Check sheet for the modelled part. Datum: model origin and axes. Units: mm. A direction names the side the tool comes from. Round coordinates to 2 decimals unless told otherwise and drop trailing zeros. Loops run counter-clockwise (first coordinate to the right, second up) from the corner with the lowest first, then second, coordinate; pieces in that order, holes last. Notation, with made-up numbers: (81, 15) - (138, 15) arc R28 ccw to (138, 42) - close; hole circle Ø4 at (79, 45.25). An arc over 180 degrees is marked (long way). Put each result on its own line as item: value.
```python
from build123d import *

# Parameters (mm, degrees)
ESQUISSE1_R             = 7.366
BOSS_EXTRU_1_DEPTH      = 9.398
BOSS_EXTRU_2_START      = -2.1844
BOSS_EXTRU_2_DEPTH      = 2.1844
CONG_1_R                = 2.54
ESQUISSE3_R             = 1.143
ENL_V_MAT_EXTRU_2_DEPTH = 16.678200152


with BuildPart() as part:
    # Esquisse1 → Boss.-Extru.1 (new body)
    with BuildSketch(Plane.XY):
        Circle(ESQUISSE1_R)
    extrude(amount=BOSS_EXTRU_1_DEPTH)

    # Esquisse2 → Boss.-Extru.2 (add)
    with BuildSketch(Plane.XY.offset(9.398).offset(BOSS_EXTRU_2_START)):
        with BuildLine():
            Line((7.366, 2.794), (6.815535195, 2.794))
            ThreePointArc((6.815535195, 2.794), (7.22707369, 1.423854584), (7.366, 0))
            Line((7.366, 0), (10.16, 0))
            ThreePointArc((10.16, 0), (9.341656347, 1.975656347), (7.366, 2.794))
        make_face()
        with BuildLine():
            Line((10.16, 0), (7.366, 0))
            ThreePointArc((7.366, 0), (7.22707369, -1.423854584), (6.815535195, -2.794))
            Line((6.815535195, -2.794), (7.366, -2.794))
            ThreePointArc((7.366, -2.794), (9.341656347, -1.975656347), (10.16, 0))
        make_face()
        with BuildLine():
            Line((-7.366, 0), (-10.16, 0))
            ThreePointArc((-10.16, 0), (-9.341656347, -1.975656347), (-7.366, -2.794))
            Line((-7.366, -2.794), (-6.815535195, -2.794))
            ThreePointArc((-6.815535195, -2.794), (-7.22707369, -1.423854584), (-7.366, 0))
        make_face()
        with BuildLine():
            Line((-6.815535195, 2.794), (-7.366, 2.794))
            ThreePointArc((-7.366, 2.794), (-9.341656347, 1.975656347), (-10.16, 0))
            Line((-10.16, 0), (-7.366, 0))
            ThreePointArc((-7.366, 0), (-7.22707369, 1.423854584), (-6.815535195, 2.794))
        make_face()
    extrude(amount=BOSS_EXTRU_2_DEPTH)

    # Congé1
    # the kernel refuses this fillet: 2.54 mm, written as the material it adds along each edge
    with BuildSketch(Plane(origin=(6.815535195, 2.794, 7.2136), x_dir=(-0.45524151464262924, 0.8903679932173465, 0), z_dir=(0, 0, 1)), Plane(origin=(-6.815535195, -2.794, 7.2136), x_dir=(0.4552415146426176, -0.8903679932173524, 0), z_dir=(0, 0, 1))) as cong_1_piece_1:
        with BuildLine():
            CenterArc((1.442130851, -2.531130754), CONG_1_R, 94.789504406, 46.813825589)
            Line((-0.548542223, -0.953531086), (-0.74760953, -0.795771119))
            ThreePointArc((-0.74760953, -0.795771119), (-0.476747902, -0.374484899), (-0.22615347, 0.115631345))
            Line((-0.22615347, 0.115631345), (0.021207807, 0.253113075))
            ThreePointArc((0.021207807, 0.253113075), (0.615026392, 0.228279187), (1.208844978, 0.253113075))
            Line((1.208844978, 0.253113075), (1.230052785, 0))
        make_face()
    extrude(amount=2.1844)
    with BuildSketch(Plane(origin=(6.815535195, -2.794, 7.2136), x_dir=(-0.4552415146426287, -0.8903679932173468, 0), z_dir=(0, 0, 1)), Plane(origin=(-6.815535195, 2.794, 7.2136), x_dir=(0.45524151464261825, 0.890367993217352, 0), z_dir=(0, 0, 1))) as cong_1_piece_2:
        with BuildLine():
            CenterArc((1.442130851, 2.531130754), CONG_1_R, 218.396670004, 46.813825589)
            Line((-0.548542223, 0.953531086), (-0.74760953, 0.795771119))
            ThreePointArc((-0.74760953, 0.795771119), (-0.476747902, 0.374484899), (-0.22615347, -0.115631345))
            Line((-0.22615347, -0.115631345), (0.021207807, -0.253113075))
            ThreePointArc((0.021207807, -0.253113075), (0.615026392, -0.228279187), (1.208844978, -0.253113075))
            Line((1.208844978, -0.253113075), (1.230052785, 0))
        make_face()
    extrude(amount=2.1844)

    # Esquisse3 → Enlèv. mat.-Extru.2 (cut, through all)
    with BuildSketch(Plane.XY.offset(9.398)):
        with Locations((-7.366, 0)):
            Circle(ESQUISSE3_R)
        with Locations((7.366, 0)):
            Circle(ESQUISSE3_R)
    extrude(amount=-ENL_V_MAT_EXTRU_2_DEPTH, mode=Mode.SUBTRACT)

    # Esquisse4 → Cut-Revolve1 (revolve, cut)
    with BuildSketch(Plane(origin=(0, 0, 0), x_dir=(0, 0, -1), z_dir=(1, 0, 0))):
        with BuildLine():
            Line((-8.4836, 0), (4.064, 0))
            ThreePointArc((4.064, 0), (-2.2098, 6.2738), (-8.4836, 0))
        make_face()
    revolve(axis=Axis((0, 0, 7.037287666), (0, 0, -1)), mode=Mode.SUBTRACT)


solid = part.part
```
Item 1: Go/stop test with flat-tipped pins: pin 1 (2 mm diameter, centred on y = 3, z = 2, fed in from -X); pin 2 (1.5 mm diameter, centred on y = 2, z = 7.5, fed in from -X); pin 3 (5 mm diameter, centred on y = -2.5, z = 6, fed in from -X). Record where each tip stops, or that it passes through.
Filled sheet:
pin 1: x = -7.09
pin 2: x = -9.86
pin 3: x = -10.14
Item 2: Release check for a two-part mould opening along Y. For faces 4 (the cylindrical face through (-6.954, -3.151, 8.291)), 5 (the cylindrical face through (-6.31, -0.44, 5.81)), 6 (the flat face through (1, 6, 0)) record: +Y half, -Y half, draft (parallel to the pull), parting line (faces both ways), or undercut.
Filled sheet:
face 4: -Y half
face 5: undercut
face 6: draft
Item 3: Section check B-B on z = 6.75. Enter the section's corners in (x, y).
Filled sheet:
outline: (-7.28, -1.14) arc R7.37 ccw to (7.28, -1.14) arc R1.14 cw to (7.28, 1.14) arc R7.37 ccw to (-7.28, 1.14) arc R1.14 cw to start; hole circle Ø8.66 at (0, 0)
Item 4: Thickness scan on line 1 (Y direction, x = 6.5, z = 1); line 2 (X direction, y = 0, z = 6); line 3 (Y direction, x = 1, z = 3.75). Record the ranges inside material, lowest first. Write a range as from..to.
Filled sheet:
line 1: -3.47..-0.75, 0.75..3.47
line 2: -6.22..-5, 5..6.22
line 3: -7.3..-6, 6..7.3
Item 5: Section check C-C on y = 4.25. Enter the section's corners in (x, z).
Filled sheet:
outline: (-6.02, 0) - (-4.05, 0) arc R4.61 cw (long way) to (4.05, 0) - (6.02, 0) - (6.02, 9.4) - (-6.02, 9.4) - close
Item 6: Tool access check on faces 1 (the cylindrical face through (-0.146, -7.365, 4.633)), 2 (the cylindrical face through (0.146, 7.365, 4.633)), 3 (the flat face through (0, 0, 9.398)). Record the directions out of +Z, -Z, +X, -X, +Y, -Y that give a thin tool (end or side, any length) a straight path to the whole face; none if there is none.
Filled sheet:
face 1: -Z, -Y
face 2: -Z, +Y
face 3: +Z, +X, -X, +Y, -Y
Item 7: Section check A-A on x = -7.5. Enter the section's corners in (y, z), then the cut area to 3 significant figures.
Filled sheet:
outline: (-2.86, 7.21) - (-1.14, 7.21) - (-1.14, 9.4) - (-2.86, 9.4) - close; (1.14, 7.21) - (2.86, 7.21) - (2.86, 9.4) - (1.14, 9.4) - close
area: 7.54 mm²
Item 8: Section check D-D on x = 2.25. Enter the section's corners in (y, z).
Filled sheet:
outline: (-7.01, 0) - (-5.42, 0) arc R5.86 cw (long way) to (5.42, 0) - (7.01, 0) - (7.01, 9.4) - (-7.01, 9.4) - close
